from build123d import *

# Parameters (mm, degrees)
F1_DEPTH = 1
F2_DEPTH = 128


with BuildPart() as f1:
    # F0 (on Front) → F1 (new body)
    with BuildSketch(Plane.XZ):
        Polygon((5, -1), (1.618034, -1), (5, -7.763932), (8.381966, -1), align=None)
    extrude(amount=F1_DEPTH)

    # F0 (on Front) → F2 (join)
    with BuildSketch(Plane.XZ):
        Polygon((5, 0), (0, 0), (5, -10), (10, 0), align=None)
        Polygon((5, -7.763932), (1.618034, -1), (5, -1), (8.381966, -1), align=None, mode=Mode.SUBTRACT)
    extrude(amount=F2_DEPTH)


solid = f1.part
Design review of the part built by this model. Coordinates are the model's own, in mm. A direction names the side the tool comes from. Round coordinates to 2 decimals unless told otherwise and drop trailing zeros. Write each loop counter-clockwise with the first axis right and the second up, starting at its lowest first coordinate (ties: lowest second). Pieces come first, ordered by that corner, then holes.
Item 1: Consider section A-A on y = -74. Give the boundary of the cut face in (x, z).
Item 2: Consider section B-B on z = -5. Give the boundary of the cut face in (x, y).
Item 3: For faces 1 (the flat face through (3.333, -63.611, -4.429)), 2 (the flat face through (7.465, -63.104, -5.07)), list the 3-axis set-ups (+Z, -Z, +X, -X, +Y, -Y) from which the entire face can be reached by the end or side of a thin tool; tool diameter is ignored.
Item 4: Consider section C-C on x = 6.75. Give the boundary of the cut face in (y, z), and give its area (3 significant figures).
Item 5: Wall thickness on L1, parallel to Z at x = 2.5, y = -23; L2, parallel to Z at x = 7.75, y = -28; L3, parallel to X at y = -33, z = -5.5: over which ranges is each line inside the solid? List them lowest first.
Item 6: For pin 1 Ø1.5 at (x, z) = (7.5, -2.5) entering from +Y; pin 2 Ø2 at (x, z) = (1.5, -8) entering from -Y; pin 3 Ø3 at (y, z) = (-60.5, -5) entering from -X; pin 4 Ø4 at (x, y) = (8.5, -72) entering from -Z, all flat-tipped, find the tip position at first contact; note any pin that passes through.
Item 7: Draft analysis for pull direction Z (two halves, no side actions). For faces 3 (the flat face through (6.715, -63.611, -4.335)), 4 (the flat face through (2.465, -63.104, -4.93)), 5 (the flat face through (5, -1, -4)), 6 (the flat face through (5, 0, -4)), state which applies: released by +Z, released by -Z, zero draft, split by the parting line, or undercut.
Check values:
1. outline: (0, 0) - (5, -10) - (10, 0) - close; hole (1.62, -1) - (5, -7.76) - (8.38, -1) - close
2. outline: (2.5, -128) - (3.62, -128) - (3.62, -1) - (6.38, -1) - (6.38, -128) - (7.5, -128) - (7.5, 0) - (2.5, 0) - close
3. face 1: -Y
3. face 2: -Z, +X, +Y, -Y
4. outline: (-128, -6.5) - (0, -6.5) - (0, 0) - (-128, 0) - (-128, -1) - (-1, -1) - (-1, -4.26) - (-128, -4.26) - close
4. area: 417 mm2
5. L1: z = -5 to -2.76, -1 to 0
5. L2: z = -4.5 to -2.26, -1 to 0
5. L3: x = 2.75 to 3.87, 6.13 to 7.25
6. pin 1: stops at y = 0
6. pin 2: passes through
6. pin 3: stops at x = 1.75
6. pin 4: stops at z = -7
7. face 3: undercut
7. face 4: released by -Z
7. face 5: undercut
7. face 6: zero draft
